Here's how the part is built. I have some questions about the finished solid (model axes, mm). Face numbers are marked on the shaded views. A direction names the side the tool comes from. Give positions to 0.01 mm unless a question says otherwise; leave off trailing zeros. Write each loop counter-clockwise with the first axis right and the second up, starting at its lowest first coordinate (ties: lowest second). Pieces come first, ordered by that corner, then holes. Notation, with made-up numbers: (9.25, -1.5) -> (44.25, -1.5) arc R28 ccw to (44.25, 30.5) -> close; hole circle Ø10 at (68, 60.25). An arc over 180 degrees is marked (long way). Return JSON: item names as keys, results as strings.
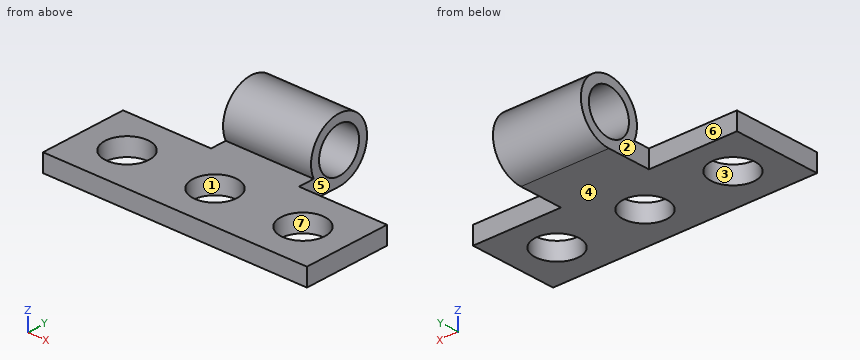
from build123d import *

# Parameters (mm, degrees)
SKETCH1_W                = 30
SKETCH1_H                = 10
BOSS_EXTRUDE1_DEPTH      = 2
SKETCH2_R                = 2.5
BOSS_EXTRUDE2_DEPTH      = 5
BOSS_EXTRUDE2_DEPTH_BACK = 5
SKETCH3_R                = 2.5
CUT_EXTRUDE1_DEPTH       = 10


with BuildPart() as part:
    # Sketch1 → Boss-Extrude1 (new body)
    with BuildSketch(Plane.XY):
        Rectangle(SKETCH1_W, SKETCH1_H)
    extrude(amount=BOSS_EXTRUDE1_DEPTH)

    # Sketch2 → Boss-Extrude2 (add, two sides)
    with BuildSketch(Plane.ZY) as boss_extrude2_sk:
        with BuildLine():
            Line((0, 5), (0, 10))
            ThreePointArc((0, 10), (6.458039892, 11.870828693), (2, 6.83772234))
            Line((2, 6.83772234), (2, 5))
            Line((2, 5), (0, 5))
        make_face()
        with Locations((3.5, 10)):
            Circle(SKETCH2_R, mode=Mode.SUBTRACT)
    extrude(amount=BOSS_EXTRUDE2_DEPTH)
    extrude(boss_extrude2_sk.sketch, amount=-BOSS_EXTRUDE2_DEPTH_BACK)

    # Sketch3 → Cut-Extrude1 (cut)
    with BuildSketch(Plane.XY.offset(2)):
        with Locations((-10, 0)):
            Circle(SKETCH3_R)
        Circle(SKETCH3_R)
        with Locations((10, 0)):
            Circle(SKETCH3_R)
    extrude(amount=-CUT_EXTRUDE1_DEPTH, mode=Mode.SUBTRACT)


solid = part.part
1. Which directions (+Z, -Z, +X, -X, +Y, -Y) give clear straight access to the entire face, cutting with the end or side of a thin tool? Please do the marked faces 5, 6 and 7.
Taken from the geometry:
{"face 5": "+Z, -Z, +X, +Y", "face 6": "+Z, -Z, -X, +Y", "face 7": "+Z, -Z"}
2. Suppose I cut it at D-D, the plane y = 1. List the corners of the cut face in (x, z) for me.
Taken from the geometry:
{"outline": "(-15, 0) -> (-12.29, 0) -> (-12.29, 2) -> (-15, 2) -> close; (-7.71, 0) -> (-2.29, 0) -> (-2.29, 2) -> (-7.71, 2) -> close; (2.29, 0) -> (7.71, 0) -> (7.71, 2) -> (2.29, 2) -> close; (12.29, 0) -> (15, 0) -> (15, 2) -> (12.29, 2) -> close"}
3. For pin 1 Ø3.5 at (x, y) = (-4, 0) entering from +Z; pin 2 Ø2 at (y, z) = (7, 4) entering from -X; pin 3 Ø2 at (x, z) = (-8, 1) entering from +Y, each with a flat end and sliding along its axis, tell me the tip position at first contact or that it passes through.
Taken from the geometry:
{"pin 1": "stops at z = 2", "pin 2": "stops at x = -5", "pin 3": "stops at y = 5"}
4. Suppose I cut it at B-B, the plane z = 3.5. List the corners of the cut face in (x, y) for me, and give its area (3 significant figures).
Taken from the geometry:
{"outline": "(-5, 6.5) -> (5, 6.5) -> (5, 7.5) -> (-5, 7.5) -> close; (-5, 12.5) -> (5, 12.5) -> (5, 13.5) -> (-5, 13.5) -> close", "area": "20.0 mm²"}
5. If I drill on line 1 (Y direction, x = 2, z = 3.5); line 2 (Y direction, x = 10, z = 1.65); line 3 (Z direction, x = 11.5, y = -2.5), over which ranges is the centre line in solid material (lowest first)? Write a range as [from, to].
Taken from the geometry:
{"line 1": "y = [6.5, 7.5], [12.5, 13.5]", "line 2": "y = [-5, -2.5], [2.5, 5]", "line 3": "z = [0, 2]"}
6. If we mould it in two halves opening along X, with no side actions, what happens to the marked faces 1, 2, 3 and 4? For each: released by +X, released by -X, zero draft, split by the parting line, or undercut.
Taken from the geometry:
{"face 1": "undercut", "face 2": "released by -X", "face 3": "undercut", "face 4": "zero draft"}
7. Suppose I cut it at C-C, the plane x = -10. List the corners of the cut face in (y, z) for me, and give its area (3 significant figures).
Taken from the geometry:
{"outline": "(-5, 0) -> (-2.5, 0) -> (-2.5, 2) -> (-5, 2) -> close; (2.5, 0) -> (5, 0) -> (5, 2) -> (2.5, 2) -> close", "area": "10.0 mm²"}
8. Suppose I cut it at A-A, the plane x = 1.5. List the corners of the cut face in (y, z) for me.
Taken from the geometry:
{"outline": "(-5, 0) -> (-2, 0) -> (-2, 2) -> (-5, 2) -> close; (2, 0) -> (10, 0) arc R3.5 ccw (long way) to (6.84, 2) -> (2, 2) -> close; hole circle Ø5 at (10, 3.5)"}
